For this review, take the finished solid that the model builds, in its own axes (mm). A direction names the side the tool comes from. Coordinates: 2 decimals unless noted, no trailing zeros. Loops run counter-clockwise (first coordinate to the right, second up) from the corner with the lowest first, then second, coordinate; pieces in that order, holes last. Notation, with made-up numbers: M 78.5,36 L 106.5,36 A20 cw 106.5,53 Z; hole C 31.25,12 d2. An arc over 180 degrees is marked long. Put each result on its own line as item: value.
```python
from build123d import *

# Parameters (mm, degrees)
BASE_EXTRUDE_DEPTH = 9.525
ARCH_EXTRUDE_DEPTH = 19.05
SKETCH3_R          = 12.7
ARCH_CUT_DEPTH     = 50.222663057
SKETCH4_R          = 7.1501
LARGE_CUT_DEPTH    = 4.191
SKETCH5_R          = 3.3782
SMALL_CUT_DEPTH    = 45.068684339


with BuildPart() as part:
    # Sketch1 → Base Extrude (new body)
    with BuildSketch(Plane(origin=(0, 0, 0), x_dir=(1, 0, 0), z_dir=(0, 1, 0))):
        with BuildLine():
            Line((-29.21, 9.525), (30.047938144, 9.525))
            ThreePointArc((30.047938144, 9.525), (39.572938144, 0), (30.047938144, -9.525))
            Line((30.047938144, -9.525), (-29.21, -9.525))
            ThreePointArc((-29.21, -9.525), (-38.735, 0), (-29.21, 9.525))
        make_face()
    extrude(amount=BASE_EXTRUDE_DEPTH)

    # Sketch2 → Arch Extrude (add)
    with BuildSketch(Plane.XY.offset(9.525)):
        with BuildLine():
            Line((-21.806030928, 0), (22.643969072, 0))
            ThreePointArc((22.643969072, 0), (22.101207406, 4.881717509), (20.499432214, 9.525))
            Line((20.499432214, 9.525), (-19.66149407, 9.525))
            ThreePointArc((-19.66149407, 9.525), (-21.263269262, 4.881717509), (-21.806030928, 0))
        make_face()
        with BuildLine():
            Line((-19.66149407, 9.525), (20.499432214, 9.525))
            ThreePointArc((20.499432214, 9.525), (0.418969072, 22.225), (-19.66149407, 9.525))
        make_face()
    extrude(amount=-ARCH_EXTRUDE_DEPTH)

    # Sketch3 → Arch Cut (cut, through all)
    with BuildSketch(Plane.XY.offset(9.525)):
        Circle(SKETCH3_R)
    extrude(amount=-ARCH_CUT_DEPTH, mode=Mode.SUBTRACT)

    # Sketch4 → Large Cut (cut)
    with BuildSketch(Plane(origin=(0, 9.525, 0), x_dir=(1, 0, 0), z_dir=(0, 1, 0))):
        with Locations(Location((-29.21, 0, 0), (0, 0, 270))):
            Circle(SKETCH4_R)
    large_cut = extrude(amount=-LARGE_CUT_DEPTH, mode=Mode.SUBTRACT)

    # Sketch5 → Small Cut (cut, through all)
    with BuildSketch(Plane(origin=(0, 5.334, 0), x_dir=(1, 0, 0), z_dir=(0, 1, 0))):
        with Locations(Location((-29.21, 0, 0), (0, 0, 270))):
            Circle(SKETCH5_R)
    small_cut = extrude(amount=-SMALL_CUT_DEPTH, mode=Mode.SUBTRACT)

    # Mirror 2: Large Cut, Small Cut across plane
    add(large_cut.mirror(Plane(origin=(0, 0, 0), x_dir=(0, 0, 1), z_dir=(1, 0, 0))), mode=Mode.SUBTRACT)
    add(small_cut.mirror(Plane(origin=(0, 0, 0), x_dir=(0, 0, 1), z_dir=(1, 0, 0))), mode=Mode.SUBTRACT)


solid = part.part
```
(1) Add section A-A (y = 2.75). Write out the cut boundary in (x, z) (3 decimals), plus the area to 3 significant figures.
Determined:
outline: M -29.21,-9.525 L -12.399,-9.525 L -12.399,9.525 L -29.21,9.525 A9.525 ccw Z; M 12.399,-9.525 L 30.048,-9.525 A9.525 ccw 30.048,9.525 L 12.399,9.525 Z; hole C -29.21,0 d6.756; hole C 29.21,0 d6.756
area: 870 mm^2
(2) Tool access review of faces 1 (the flat face through (27.5, 5.334, 3.1)), 2 (the flat face through (-23, 9.525, -4)), 3 (the flat face through (37, 9.525, 0)): name each direction out of +Z, -Z, +X, -X, +Y, -Y from which nothing blocks a thin tool from reaching the whole face with its end or side.
Determined:
face 1: +Y
face 2: +Z, -Z, -X, +Y
face 3: +Z, -Z, +X, +Y
(3) Add section D-D (x = 27.5). Write out the cut boundary in (y, z) (3 decimals).
Determined:
outline: M 0,-9.525 L 9.525,-9.525 L 9.525,-6.943 L 5.334,-6.943 L 5.334,-2.913 L 0,-2.913 Z; M 0,2.913 L 5.334,2.913 L 5.334,6.943 L 9.525,6.943 L 9.525,9.525 L 0,9.525 Z
(4) Wall thickness on line 1 along Z through (x, y) = (29.21, 1.3) (3 decimals); line 2 along X through (y, z) = (8.05, 0) (3 decimals); line 3 along X through (y, z) = (7.2, 0) (3 decimals): over which ranges is each line inside the solid? List them lowest first. Write a range as [from, to].
Determined:
line 1: z = [-9.525, -3.378], [3.378, 9.525]
line 2: x = [-38.735, -36.36], [-22.06, -9.823], [9.823, 22.06], [36.36, 39.573]
line 3: x = [-38.735, -36.36], [-22.06, -10.462], [10.462, 22.06], [36.36, 39.573]
(5) Add section C-C (x = -28). Write out the cut boundary in (y, z) (3 decimals).
Determined:
outline: M 0,-9.525 L 9.525,-9.525 L 9.525,-7.047 L 5.334,-7.047 L 5.334,-3.154 L 0,-3.154 Z; M 0,3.154 L 5.334,3.154 L 5.334,7.047 L 9.525,7.047 L 9.525,9.525 L 0,9.525 Z
(6) For pin 1 (8 mm diameter, centred on x = 29.21, z = 0, fed in from +Y); pin 2 (1.5 mm diameter, centred on x = 26, y = 10, fed in from -Z) (3 decimals); pin 3 (9.5 mm diameter, centred on x = -26.5, z = 3.5, fed in from +Y) (3 decimals), all flat-tipped, find the tip position at first contact; note any pin that passes through.
Determined:
pin 1: stops at y = 5.33
pin 2: stops at z = -9.525
pin 3: stops at y = 9.525
(7) Add section B-B (z = 0). State how many separate pieces and enclosed holes the cut face has, plus the area to 3 significant figures.
Determined:
separate pieces: 3
enclosed holes: 0
area: 666 mm^2
(8) Draft analysis for pull direction Z (two halves, no side actions). For faces 4 (the cylindrical face through (32.51, 2.7, -0.73)), 5 (the cylindrical face through (-22.12, 7.46, -0.93)), 6 (the flat face through (1, 13, 9.525)), 7 (the flat face through (-23, 0, 0)), state which applies: +Z half, -Z half, draft (parallel to the pull), parting line (faces both ways), or undercut.
Determined:
face 4: undercut
face 5: undercut
face 6: +Z half
face 7: draft
